Verification items for the finished model (mm, model axes). A direction names the side the tool comes from. Coordinates: 2 decimals unless noted, no trailing zeros. Loops run counter-clockwise (first coordinate to the right, second up) from the corner with the lowest first, then second, coordinate; pieces in that order, holes last. Notation, with made-up numbers: (81, 30) -> (100, 30) arc R24 cw to (100, 59) -> close; hole circle Ø8 at (-37, -20.5). An arc over 180 degrees is marked (long way). Answer as a JSON object with one key per item and string values. Group by question number.
Q1. Cross-section at D-D on y = -2.75. Record the boundary of the cut face in (x, z), and give its area (3 significant figures).
Q2. Cross-section at A-A on x = 2.5. Record the boundary of the cut face in (y, z), and give its area (3 significant figures).
Q3. Cross-section at C-C on z = -1.65. Record the boundary of the cut face in (x, y).
Q4. Scan lines: L1, parallel to Z at x = -5, y = -1.5; L2, parallel to Z at x = 0.5, y = -1.5; L3, parallel to Y at x = -2, z = -0.95. Record each from-to range of solid material in increasing order.
Q5. Cross-section at B-B on y = -2.1. Record the boundary of the cut face in (x, z).
Q6. Set-up check for faces 1 (the flat face through (3, -1, -2.55)), 2 (the flat face through (0, -1, 2.75)): record each of +Z, -Z, +X, -X, +Y, -Y from which the full face is reachable in a straight line by a thin tool's end or side.
```python
from build123d import *

# Parameters (mm, degrees)
SKETCH2_W              = 14
SKETCH2_H              = 5.5
BOSS_EXTRUDE1_DEPTH    = 0.1
SKETCH3_W              = 14
SKETCH3_H              = 3.5
BOSS_EXTRUDE2_DEPTH    = 0.2
CONVERT_SOLID1_START   = -7
CONVERT_SOLID1_DEPTH   = 14
CONVERT_SOLID1_2_DEPTH = 14
CUT_EXTRUDE1_REACH     = 11.529
SKETCH8_W              = 2
SKETCH8_H              = 1.5
CUT_EXTRUDE2_REACH     = 11.529
SKETCH9_W              = 8.7
SKETCH9_H              = 1.8
SKETCH9_W_2            = 1.7
SKETCH9_H_2            = 1.1
SKETCH9_W_3            = 2
CUT_EXTRUDE3_REACH     = 10.295


# Read off the part's stored shape, not the designer's step: Convert-Solid1
with BuildPart() as part:
    # Sketch2 → Boss-Extrude1 (new, symmetric)
    with BuildSketch(Plane(origin=(0, 0, 0), x_dir=(1, 0, 0), z_dir=(0, 1, 0))):
        Rectangle(SKETCH2_W, SKETCH2_H)
    extrude(amount=BOSS_EXTRUDE1_DEPTH, both=True)

    # Sketch3 → Boss-Extrude2 (add)
    with BuildSketch(Plane.XY.offset(2.75)):
        with Locations((0, -1.65)):
            Rectangle(SKETCH3_W, SKETCH3_H)
    boss_extrude2 = extrude(amount=-BOSS_EXTRUDE2_DEPTH)

    # Mirror1: Boss-Extrude2 across plane
    add(boss_extrude2.mirror(Plane.XY))

    # Convert-Solid1 outline → Convert-Solid1 (cut)
    with BuildSketch(Plane.YZ.offset(CONVERT_SOLID1_START)):
        with BuildLine():
            Line((0.1, 2.75), (-0.2, 2.75))
            ThreePointArc((-0.2, 2.75), (0.012132034, 2.662132034), (0.1, 2.45))
            Line((0.1, 2.45), (0.1, 2.75))
        make_face()
        with BuildLine():
            Line((0.1, -2.75), (0.1, -2.45))
            ThreePointArc((0.1, -2.45), (0.012132034, -2.662132034), (-0.2, -2.75))
            Line((-0.2, -2.75), (0.1, -2.75))
        make_face()
    extrude(amount=CONVERT_SOLID1_DEPTH, mode=Mode.SUBTRACT)

    # Convert-Solid1 2 outline → Convert-Solid1 2 (add)
    with BuildSketch(Plane.YZ.offset(CONVERT_SOLID1_START)):
        with BuildLine():
            Line((-0.1, 2.55), (-0.2, 2.55))
            ThreePointArc((-0.2, 2.55), (-0.129289322, 2.520710678), (-0.1, 2.45))
            Line((-0.1, 2.45), (-0.1, 2.55))
        make_face()
        with BuildLine():
            Line((-0.1, -2.55), (-0.1, -2.45))
            ThreePointArc((-0.1, -2.45), (-0.129289322, -2.520710678), (-0.2, -2.55))
            Line((-0.2, -2.55), (-0.1, -2.55))
        make_face()
    extrude(amount=CONVERT_SOLID1_2_DEPTH)

    # Sketch8 → Cut-Extrude1 (cut, up to next)
    with BuildSketch(Plane.XY.offset(2.75), mode=Mode.PRIVATE) as cut_extrude1_sk1:
        Polygon((-4.2, -3.4), (-4.2, -1.9), (-3.4, -1.9), (-3.4, -1.4), (5, -1.4), (5, -2.4), (6.2, -2.4), (6.2, -3.4), align=None)
    cut_extrude1_tool1 = extrude(cut_extrude1_sk1.sketch, amount=-CUT_EXTRUDE1_REACH, mode=Mode.PRIVATE) & part.part
    # Sketch8 → Cut-Extrude1 (cut, up to next)
    with BuildSketch(Plane.XY.offset(2.75), mode=Mode.PRIVATE) as cut_extrude1_sk2:
        with Locations((-6, -2.65)):
            Rectangle(SKETCH8_W, SKETCH8_H)
    cut_extrude1_tool2 = extrude(cut_extrude1_sk2.sketch, amount=-CUT_EXTRUDE1_REACH, mode=Mode.PRIVATE) & part.part
    add(cut_extrude1_tool1.solids().sort_by_distance((0.8125, -2.446875, 2.75))[0], mode=Mode.SUBTRACT)
    add(cut_extrude1_tool2.solids().sort_by_distance((-6, -2.65, 2.75))[0], mode=Mode.SUBTRACT)

    # Sketch9 → Cut-Extrude2 (cut, up to next)
    with BuildSketch(Plane(origin=(0, 0, -2.75), x_dir=(-1, 0, 0), z_dir=(0, 0, -1)), mode=Mode.PRIVATE) as cut_extrude2_sk1:
        with Locations((-2.65, -2.5)):
            Rectangle(SKETCH9_W, SKETCH9_H)
    cut_extrude2_tool1 = extrude(cut_extrude2_sk1.sketch, amount=-CUT_EXTRUDE2_REACH, mode=Mode.PRIVATE) & part.part
    # Sketch9 → Cut-Extrude2 (cut, up to next)
    with BuildSketch(Plane(origin=(0, 0, -2.75), x_dir=(-1, 0, 0), z_dir=(0, 0, -1)), mode=Mode.PRIVATE) as cut_extrude2_sk2:
        with Locations((3.35, -2.85)):
            Rectangle(SKETCH9_W_2, SKETCH9_H_2)
    cut_extrude2_tool2 = extrude(cut_extrude2_sk2.sketch, amount=-CUT_EXTRUDE2_REACH, mode=Mode.PRIVATE) & part.part
    # Sketch9 → Cut-Extrude2 (cut, up to next)
    with BuildSketch(Plane(origin=(0, 0, -2.75), x_dir=(-1, 0, 0), z_dir=(0, 0, -1)), mode=Mode.PRIVATE) as cut_extrude2_sk3:
        with Locations((6, -2.85)):
            Rectangle(SKETCH9_W_3, SKETCH9_H_2)
    cut_extrude2_tool3 = extrude(cut_extrude2_sk3.sketch, amount=-CUT_EXTRUDE2_REACH, mode=Mode.PRIVATE) & part.part
    add(cut_extrude2_tool1.solids().sort_by_distance((2.65, -2.5, -2.75))[0], mode=Mode.SUBTRACT)
    add(cut_extrude2_tool2.solids().sort_by_distance((-3.35, -2.85, -2.75))[0], mode=Mode.SUBTRACT)
    add(cut_extrude2_tool3.solids().sort_by_distance((-6, -2.85, -2.75))[0], mode=Mode.SUBTRACT)

    # Sketch10 → Cut-Extrude3 (cut, up to next)
    with BuildSketch(Plane(origin=(0, 0.1, 0), x_dir=(1, 0, 0), z_dir=(0, 1, 0)), mode=Mode.PRIVATE) as cut_extrude3_sk1:
        Polygon((-1.7, -1.45), (5.4, -1.45), (5.4, 0.25), (4.4, 0.25), (4.4, -0.45), (-0.7, -0.45), (-0.7, 2.75), (-1.7, 2.75), align=None)
    cut_extrude3_tool1 = extrude(cut_extrude3_sk1.sketch, amount=-CUT_EXTRUDE3_REACH, mode=Mode.PRIVATE) & part.part
    add(cut_extrude3_tool1.solids().sort_by_distance((1.85, 0.1, 1.367508))[0], mode=Mode.SUBTRACT)


solid = part.part
```
Computed values:
{
 "1": {"outline": "(-5, -2.75) -> (-4.2, -2.75) -> (-4.2, -2.55) -> (-5, -2.55) -> close; (-5, 2.55) -> (-4.2, 2.55) -> (-4.2, 2.75) -> (-5, 2.75) -> close; (-2.5, -2.75) -> (-1.7, -2.75) -> (-1.7, -2.55) -> (-2.5, -2.55) -> close; (6.2, 2.55) -> (7, 2.55) -> (7, 2.75) -> (6.2, 2.75) -> close", "area": "0.640 mm²"},
 "2": {"outline": "(-1.6, -2.75) -> (-0.2, -2.75) arc R0.3 ccw to (0.1, -2.45) -> (0.1, 0.45) -> (-0.1, 0.45) -> (-0.1, -2.45) arc R0.1 cw to (-0.2, -2.55) -> (-1.6, -2.55) -> close; (-1.4, 2.55) -> (-0.2, 2.55) arc R0.1 cw to (-0.1, 2.45) -> (-0.1, 1.45) -> (0.1, 1.45) -> (0.1, 2.45) arc R0.3 ccw to (-0.2, 2.75) -> (-1.4, 2.75) -> close", "area": "1.43 mm²"},
 "3": {"outline": "(-7, -0.1) -> (-1.7, -0.1) -> (-1.7, 0.1) -> (-7, 0.1) -> close; (-0.7, -0.1) -> (7, -0.1) -> (7, 0.1) -> (-0.7, 0.1) -> close"},
 "4": {"L1": "z = -2.75 to -2.55, 2.55 to 2.75", "L2": "z = -2.75 to -2.55", "L3": "y = -0.1 to 0.1"},
 "5": {"outline": "(-7, -2.75) -> (-1.7, -2.75) -> (-1.7, -2.55) -> (-7, -2.55) -> close; (-5, 2.55) -> (-4.2, 2.55) -> (-4.2, 2.75) -> (-5, 2.75) -> close; (5, 2.55) -> (7, 2.55) -> (7, 2.75) -> (5, 2.75) -> close"},
 "6": {"face 1": "+X, -X, -Y", "face 2": "+Z, +X, -X, +Y, -Y"}
}
